Could you check a few things on this model? Use its own coordinates, in mm. Face numbers are marked on the shaded views. A direction names the side the tool comes from. Coordinates: 2 decimals unless noted, no trailing zeros. Order: outer loops, then holes, each group sorted by start corner. A loop starts at its lowest first (then second) coordinate and runs counter-clockwise, first axis right, second up. Notation, with made-up numbers: (18, 85) -> (66, 85) arc R10 ccw to (66, 92) -> close; hole circle Ø5 at (2.5, 60). An arc over 180 degrees is marked (long way). Use a Markdown table: item, result. Add a question column.
1) Which directions (+Z, -Z, +X, -X, +Y, -Y) give clear straight access to the entire face, cutting with the end or side of a thin tool? Please do the marked faces 1 and 2.
2) Will these pins go through, and if not, where does the flat tip stop? pin 1 Ø1 at (x, y) = (23.5, 6.5) entering from -Z; pin 2 Ø5 at (x, z) = (24.5, 6) entering from +Y; pin 3 Ø10.5 at (x, y) = (30.5, 12) entering from +Z; pin 4 Ø3.5 at (x, z) = (25.4, 5.075) entering from +Y.
3) If I drill on L1, parallel to Z at x = 25.4, y = 1.25 (3 decimals); L2, parallel to Z at x = 43, y = 10.5; L3, parallel to Z at x = 16.5, y = 1, over which ranges is the centre line in solid material (lowest first)? Write a range as [from, to].
4) If we section it at D-D (x = 10.5): Write out the boundary of the cut face in (y, z), plus the area to 3 significant figures.
5) If we section it at C-C (x = 20): Write out the boundary of the cut face in (y, z), plus the area to 3 significant figures.
6) If we section it at A-A (x = 25.4): Write out the boundary of the cut face in (y, z) (3 decimals).
7) If we section it at B-B (y = 15.75): Write out the boundary of the cut face in (x, z).
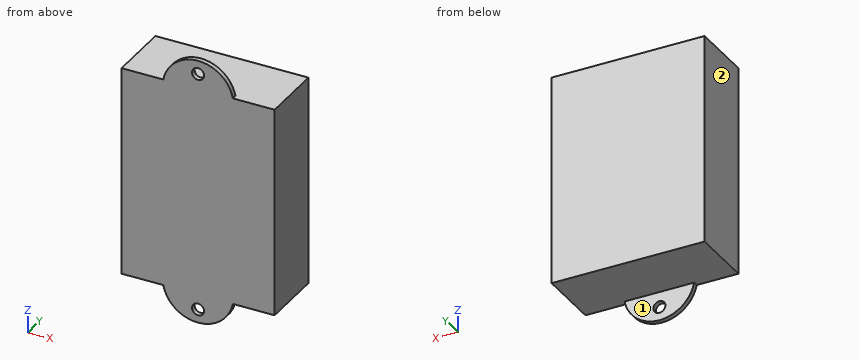
```python
from build123d import *

# Parameters (mm, degrees)
SKETCH1_W           = 50.8
SKETCH1_H           = 69.85
BOSS_EXTRUDE1_DEPTH = 21
BOSS_EXTRUDE2_DEPTH = 1.6
SKETCH3_R           = 2
CUT_EXTRUDE1_DEPTH  = 2.6


with BuildPart() as part:
    # Sketch1 → Boss-Extrude1 (new body)
    with BuildSketch(Plane(origin=(0, 0, 0), x_dir=(1, 0, 0), z_dir=(0, 1, 0))):
        with Locations((25.4, 34.925)):
            Rectangle(SKETCH1_W, SKETCH1_H)
    extrude(amount=BOSS_EXTRUDE1_DEPTH)

    # Sketch2 → Boss-Extrude2 (add)
    with BuildSketch(Plane.XZ):
        with BuildLine():
            Line((37.15368799, -2.17868799), (37.15368799, -67.67131201))
            ThreePointArc((37.15368799, -67.67131201), (25.4, -79.425), (13.64631201, -67.67131201))
            Line((13.64631201, -67.67131201), (13.64631201, -2.17868799))
            ThreePointArc((13.64631201, -2.17868799), (25.4, 9.575), (37.15368799, -2.17868799))
        make_face()
    extrude(amount=-BOSS_EXTRUDE2_DEPTH)

    # Sketch3 → Cut-Extrude1 (cut, through all)
    with BuildSketch(Plane(origin=(0, 1.6, 0), x_dir=(1, 0, 0), z_dir=(0, 1, 0))):
        with Locations((25.4, 74.925)):
            Circle(SKETCH3_R)
        with Locations((25.4, -5.075)):
            Circle(SKETCH3_R)
    extrude(amount=-CUT_EXTRUDE1_DEPTH, mode=Mode.SUBTRACT)


solid = part.part
```
Answer sheet:
| question | item | result |
|---|---|---|
| 1 | face 1 | -Z, +X, -X, +Y |
| 1 | face 2 | +Z, -Z, -X, +Y, -Y |
| 2 | pin 1 | z = -69.85 |
| 2 | pin 2 | y = 1.6 |
| 2 | pin 3 | z = 0 |
| 2 | pin 4 | through |
| 3 | L1 | [-79.425, -76.925], [-72.925, 3.075], [7.075, 9.575] |
| 3 | L2 | [-69.85, 0] |
| 3 | L3 | [-75.35, 5.5] |
| 4 | outline | (0, -69.85) -> (21, -69.85) -> (21, 0) -> (0, 0) -> close |
| 4 | area | 1,470 mm2 |
| 5 | outline | (0, -78.11) -> (1.6, -78.11) -> (1.6, -69.85) -> (21, -69.85) -> (21, 0) -> (1.6, 0) -> (1.6, 8.26) -> (0, 8.26) -> close |
| 5 | area | 1,490 mm2 |
| 6 | outline | (0, -79.425) -> (1.6, -79.425) -> (1.6, -76.925) -> (0, -76.925) -> close; (0, -72.925) -> (1.6, -72.925) -> (1.6, -69.85) -> (21, -69.85) -> (21, 0) -> (1.6, 0) -> (1.6, 3.075) -> (0, 3.075) -> close; (0, 7.075) -> (1.6, 7.075) -> (1.6, 9.575) -> (0, 9.575) -> close |
| 7 | outline | (0, -69.85) -> (50.8, -69.85) -> (50.8, 0) -> (0, 0) -> close |
